CAD build for the part. Positions are in the model's coordinates, mm. A direction names the side the tool comes from. Give positions to 0.01 mm unless a question says otherwise; leave off trailing zeros. Order: outer loops, then holes, each group sorted by start corner. A loop starts at its lowest first (then second) coordinate and runs counter-clockwise, first axis right, second up.
from build123d import *

# Parameters (mm, degrees)
F1_DEPTH = 11.1125
F2_R     = 7.9375
F3_DEPTH = 25.4
F5_DEPTH = 11.1125
F6_W     = 33.3375
F6_H     = 11.1125
F7_DEPTH = 11.1125


with BuildPart() as f1:
    # F0 (on Front) → F1 (new body)
    with BuildSketch(Plane.XZ):
        Polygon((-63.399741, 36.479078), (-95.149741, 36.479078), (-95.149741, -23.845922), (19.150259, -23.845922), (19.150259, 14.359872), align=None)
    extrude(amount=F1_DEPTH)

    # F2 (on face) → F3 (cut)
    with BuildSketch(Plane.XZ.offset(11.1125)):
        with Locations((0.100259, -4.795922)):
            Circle(F2_R)
    extrude(amount=-F3_DEPTH, mode=Mode.SUBTRACT)

    # F4 (on face) → F5 (join)
    with BuildSketch(Plane(origin=(0, 0, -23.845922), x_dir=(1, 0, 0), z_dir=(0, 0, -1))):
        Polygon((-31.649741, 11.1125), (-84.037241, 44.45), (-84.037241, 11.1125), align=None)
    extrude(amount=-F5_DEPTH)

    # F6 (on face) → F7 (join)
    with BuildSketch(Plane(origin=(-84.037241, 0, 0), x_dir=(0, -1, 0), z_dir=(-1, 0, 0))):
        with Locations((27.78125, -18.289672)):
            Rectangle(F6_W, F6_H)
        Polygon((11.1125, -12.733422), (44.45, -12.733422), (44.45, -1.620922), (27.952216, 26.954078), (11.1125, 26.954078), align=None)
    extrude(amount=F7_DEPTH)


solid = f1.part
1. 3-axis set-ups, long thin cutter, end or side, ignore diameter. For faces 1 (the flat face through (-79, -5, 36.479)), 2 (the flat face through (-90, -20, 26.954)), 3 (the flat face through (-84.037, -24, 7)): which of +Z, -Z, +X, -X, +Y, -Y reach the whole face in a straight line?
2. Saw through at A-A on x = -88. Give the cut face in (y, z).
3. Saw through at C-C on y = -36. Give the cut face in (x, z), plus the area to 3 significant figures.
4. Pin check, flat tips, straight feed: P1, Ø3, axis at x = -64, y = -26.5, coming from the +Z side; P2, Ø5, axis at x = -26.5, z = 23, coming from the +Y side; P3, Ø12, axis at x = -88.5, y = -22.5, coming from the +Z side. Stop position of each tip, or through.
5. Saw through at D-D on x = -14.5. Give the cut face in (y, z).
6. Saw through at B-B on z = -18.5. Give the cut face in (x, y), plus the area to 3 significant figures.
7. Wall check: line 1 (X direction, y = -23, z = -12); line 2 (Y direction, x = -17, z = 13.5); line 3 (Z direction, x = -66.5, y = -25). Give the ranges that are in metal, low to high.
Reported:
1. face 1: +Z, +X, -X, +Y, -Y
1. face 2: +Z, +X, -X, -Y
1. face 3: +Z, +X, -Y
2. outline: (-44.45, -23.85) - (0, -23.85) - (0, 36.48) - (-11.11, 36.48) - (-11.11, 26.95) - (-27.95, 26.95) - (-44.45, -1.62) - close
3. outline: (-95.15, -23.85) - (-70.76, -23.85) - (-70.76, -12.73) - (-84.04, -12.73) - (-84.04, 13.01) - (-95.15, 13.01) - close
3. area: 557 mm2
4. P1: stops at z = -12.73
4. P2: stops at y = 0
4. P3: stops at z = 26.95
5. outline: (-11.11, -23.85) - (0, -23.85) - (0, 23.38) - (-11.11, 23.38) - close
6. outline: (-95.15, -44.45) - (-84.04, -44.45) - (-31.65, -11.11) - (19.15, -11.11) - (19.15, 0) - (-95.15, 0) - close
6. area: 2,510 mm2
7. line 1: x = -95.15 to -84.04
7. line 2: y = -11.11 to 0
7. line 3: z = -23.85 to -12.73
